Source: CAD feature listing. Evaluate the final solid. Frame: model axes, mm. Face numbers are marked on the shaded views. A direction names the side the tool comes from. Give positions to 0.01 mm unless a question says otherwise; leave off trailing zeros. Loops run counter-clockwise (first coordinate to the right, second up) from the corner with the lowest first, then second, coordinate; pieces in that order, holes last. Notation, with made-up numbers: M 3,33.5 L 51,33.5 A27 cw 51,69.5 Z; hole C 1.25,10 d6. An arc over 180 degrees is marked long. Answer in a Markdown table with one row per item.
```python
from build123d import *

# Parameters (mm, degrees)
SKETCH4_W           = 79.375
SKETCH4_H           = 79.375
BOSS_EXTRUDE3_DEPTH = 6.35
SKETCH5_W           = 79.375
SKETCH5_H           = 79.375
SKETCH5_W_2         = 66.675
SKETCH5_H_2         = 66.675
BOSS_EXTRUDE4_DEPTH = 152.4
SKETCH7_W           = 25.4
SKETCH7_H           = 82.55
CUT_EXTRUDE1_DEPTH  = 6.35
SKETCH8_R           = 1.5875
BOSS_EXTRUDE5_DEPTH = 73.025


with BuildPart() as part:
    # Sketch4 → Boss-Extrude3 (new body)
    with BuildSketch(Plane(origin=(0, 0, 0), x_dir=(1, 0, 0), z_dir=(0, 1, 0))):
        Rectangle(SKETCH4_W, SKETCH4_H)
    extrude(amount=BOSS_EXTRUDE3_DEPTH)

    # Sketch5 → Boss-Extrude4 (add)
    with BuildSketch(Plane(origin=(0, 6.35, 0), x_dir=(1, 0, 0), z_dir=(0, 1, 0))):
        Rectangle(SKETCH5_W, SKETCH5_H)
        Rectangle(SKETCH5_W_2, SKETCH5_H_2, mode=Mode.SUBTRACT)
    extrude(amount=BOSS_EXTRUDE4_DEPTH)

    # Sketch7 → Cut-Extrude1 (cut)
    with BuildSketch(Plane(origin=(39.6875, 0, 0), x_dir=(0, 0, -1), z_dir=(1, 0, 0))):
        with Locations((0, 47.625)):
            Rectangle(SKETCH7_W, SKETCH7_H)
    extrude(amount=-CUT_EXTRUDE1_DEPTH, mode=Mode.SUBTRACT)

    # Sketch8 → Boss-Extrude5 (add)
    with BuildSketch(Plane(origin=(-33.3375, 0, 0), x_dir=(0, 0, -1), z_dir=(1, 0, 0))):
        with Locations(Location((-6.35, 63.5, 0), (0, 0, 180))):
            Circle(SKETCH8_R)
        with Locations(Location((6.35, 63.5, 0), (0, 0, 180))):
            Circle(SKETCH8_R)
    extrude(amount=BOSS_EXTRUDE5_DEPTH)


solid = part.part
```
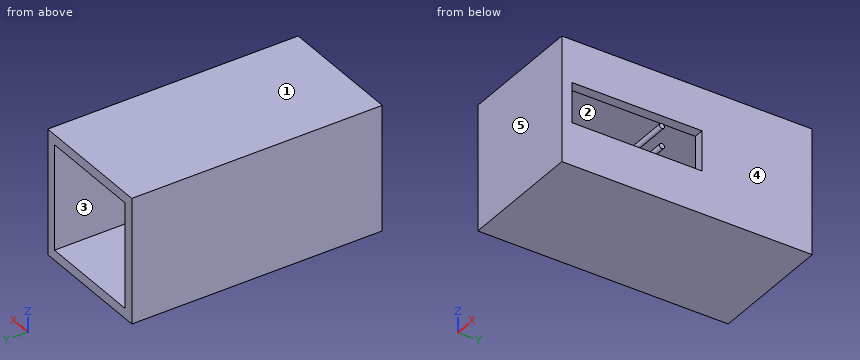
1) Section D-D, the plane y = 78.5. Return loops of the section in (x, z), then the cut area to 3 significant figures.
Reply:
| item | result |
|---|---|
| outline | M -39.69,-39.69 L 39.69,-39.69 L 39.69,-12.7 L 33.34,-12.7 L 33.34,-33.34 L -33.34,-33.34 L -33.34,33.34 L 33.34,33.34 L 33.34,12.7 L 39.69,12.7 L 39.69,39.69 L -39.69,39.69 Z |
| area | 1,690 mm² |
2) Pull-direction query (X, two-part tool) for the marked faces 3, 4 and 5; classes: released by +X, released by -X, zero draft, split by the parting line, or undercut.
Reply:
| item | result |
|---|---|
| face 3 | undercut |
| face 4 | released by +X |
| face 5 | zero draft |
3) Section B-B, the plane z = -6.35. Return loops of the section in (x, y), then the cut area to 3 significant figures.
Reply:
| item | result |
|---|---|
| outline | M -39.69,0 L 39.69,0 L 39.69,6.35 L -33.34,6.35 L -33.34,61.91 L 39.69,61.91 L 39.69,65.09 L -33.34,65.09 L -33.34,158.75 L -39.69,158.75 Z; M 33.34,88.9 L 39.69,88.9 L 39.69,158.75 L 33.34,158.75 Z |
| area | 2,150 mm² |
4) Material intervals for L1, parallel to X at y = 125, z = 11; L2, parallel to Y at x = 26.5, z = -31, sorted ascending.
Reply:
| item | result |
|---|---|
| L1 | x = -39.69 to -33.34, 33.34 to 39.69 |
| L2 | y = 0 to 6.35 |
5) Section C-C, the plane x = -27. Count the separate pieces of the cut face and the enclosed holes in it, then the cut area to 3 significant figures.
Reply:
| item | result |
|---|---|
| separate pieces | 3 |
| enclosed holes | 0 |
| area | 2,460 mm² |
6) Section A-A, the plane y = 136.5. Return loops of the section in (x, z).
Reply:
| item | result |
|---|---|
| outline | M -39.69,-39.69 L 39.69,-39.69 L 39.69,39.69 L -39.69,39.69 Z; hole M -33.34,-33.34 L 33.34,-33.34 L 33.34,33.34 L -33.34,33.34 Z |
7) Pin query (flat end, axial travel): pin 1 Ø5 at (x, z) = (35.5, 4.5) entering from -Y; pin 2 Ø3 at (x, z) = (-14, 13.5) entering from +Y; pin 3 Ø3 at (x, z) = (-8, 3.5) entering from +Y; pin 4 Ø3 at (x, z) = (-17.5, 23.5) entering from +Y. Return the tip coordinate at first contact, or that it passes through.
Reply:
| item | result |
|---|---|
| pin 1 | stops at y = 0 |
| pin 2 | stops at y = 6.35 |
| pin 3 | stops at y = 64.34 |
| pin 4 | stops at y = 6.35 |
8) Set-up query: the marked faces 1 and 2. Return all of +Z, -Z, +X, -X, +Y, -Y with unobstructed straight access to the full face (end or side cutting, diameter ignored); none if empty.
Reply:
| item | result |
|---|---|
| face 1 | +Z, +X, -X, +Y, -Y |
| face 2 | +Y |
